The drawing under review shows one solid part. Ordinate dimensions are in mm from its lowest x, y, z. A direction names the side the tool comes from. Round coordinates to 2 decimals unless told otherwise and drop trailing zeros. Write each loop counter-clockwise with the first axis right and the second up, starting at its lowest first coordinate (ties: lowest second). Pieces come first, ordered by that corner, then holes. Notation, with made-up numbers: (35.5, 18) -> (63.5, 18) arc R11 ccw to (63.5, 26) -> close; hole circle Ø4 at (22.5, -5.75). An arc over 180 degrees is marked (long way). Answer in a Markdown table with one row per item.
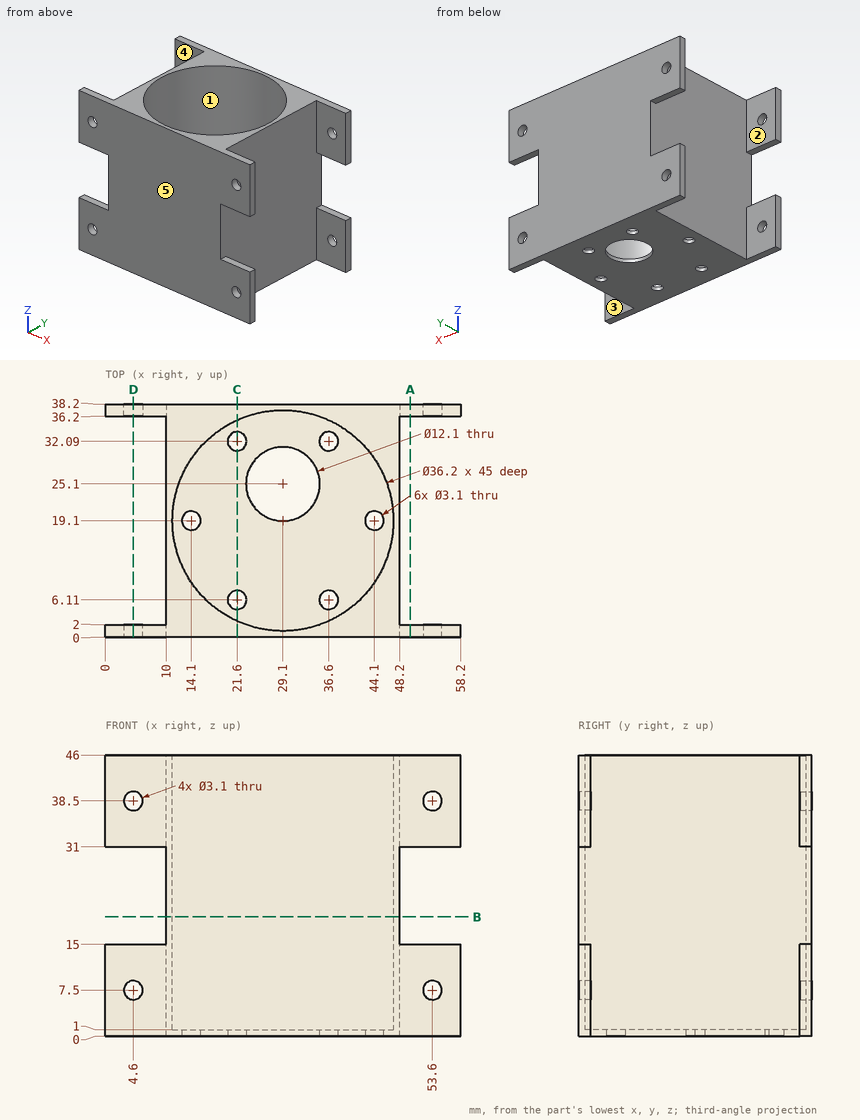
1) Mouldability with a two-part tool opening along X and no side actions: class the marked faces 1 and 2 as pulls with the +X half, pulls with the -X half, needs draft (parallel to the pull), parting line crosses it, or undercut.
Solved:
| item | result |
|---|---|
| face 1 | undercut |
| face 2 | needs draft |
2) Consider section D-D on x = 4.6. State how many separate pieces and enclosed holes the cut face has.
Solved:
| item | result |
|---|---|
| separate pieces | 8 |
| enclosed holes | 0 |
3) For line 1 (Z direction, x = 53.6, y = 1.15); line 2 (Y direction, x = 54, z = 10); line 3 (Y direction, x = 29.5, z = 6) (1 decimal), list the stretches that pass through material, from the lowest coordinate up. Write a range as [from, to].
Solved:
| item | result |
|---|---|
| line 1 | [0, 5.95], [9.05, 15], [31, 36.95], [40.05, 46] |
| line 2 | [0, 2], [36.2, 38.2] |
| line 3 | [0, 1], [37.2, 38.2] |
4) Consider section A-A on x = 50. State the section outline as (y, z) points.
Solved:
| item | result |
|---|---|
| outline | (0, 0) -> (2, 0) -> (2, 15) -> (0, 15) -> close; (0, 31) -> (2, 31) -> (2, 46) -> (0, 46) -> close; (36.2, 0) -> (38.2, 0) -> (38.2, 15) -> (36.2, 15) -> close; (36.2, 31) -> (38.2, 31) -> (38.2, 46) -> (36.2, 46) -> close |
5) Consider section B-B on z = 19.5. State the section outline as (x, y) points.
Solved:
| item | result |
|---|---|
| outline | (10, 0) -> (48.2, 0) -> (48.2, 38.2) -> (10, 38.2) -> close; hole circle Ø36.2 at (29.1, 19.1) |
6) Clearance check with flat-ended pins moving along their axes: pin 1 Ø10 at (y, z) = (24.5, 26) entering from -X; pin 2 Ø2 at (x, y) = (37.5, 7.5) entering from +Z; pin 3 Ø11.5 at (y, z) = (16, 28.5) entering from +X. State where each tip first meets the part, or that it passes through.
Solved:
| item | result |
|---|---|
| pin 1 | x = 10 |
| pin 2 | z = 1 |
| pin 3 | x = 48.2 |
7) Consider section C-C on x = 21.6. State the section outline as (y, z) points.
Solved:
| item | result |
|---|---|
| outline | (0, 0) -> (4.56, 0) -> (4.56, 1) -> (2.63, 1) -> (2.63, 46) -> (0, 46) -> close; (7.66, 0) -> (30.54, 0) -> (30.54, 1) -> (7.66, 1) -> close; (33.64, 0) -> (38.2, 0) -> (38.2, 46) -> (35.57, 46) -> (35.57, 1) -> (33.64, 1) -> close |
8) For the marked faces 3, 4 and 5, list the 3-axis set-ups (+Z, -Z, +X, -X, +Y, -Y) from which the entire face can be reached by the end or side of a thin tool; tool diameter is ignored.
Solved:
| item | result |
|---|---|
| face 3 | +Z, -Z, +X |
| face 4 | +Z, -Z, -X |
| face 5 | +Z, -Z, +X, -X, -Y |
